Could you check a few things on this drawing? It's one solid part, dimensions in mm from its lowest x, y, z. A direction names the side the tool comes from. Coordinates: 2 decimals unless noted, no trailing zeros. Order: outer loops, then holes, each group sorted by start corner. A loop starts at its lowest first (then second) coordinate and runs counter-clockwise, first axis right, second up. Notation, with made-up numbers: (41.5, -31) - (63.5, -31) arc R19 ccw to (63.5, -13) - close; hole circle Ø10 at (62.5, -20). An arc over 180 degrees is marked (long way). Answer in a Markdown table with one row per item. Add a question column.
Item 1: I want a section at D-D (x = 37.5). Please give me the cut outline in (y, z).
Item 2: Will these pins go through, and if not, where does the flat tip stop? pin 1 Ø5 at (y, z) = (94.5, 3) entering from +X; pin 2 Ø5 at (x, z) = (37.5, 6) entering from -Y; pin 3 Ø2.5 at (x, y) = (125.38, 45.19) entering from -Z; pin 4 Ø8 at (x, y) = (75.5, 97.5) entering from -Z.
Item 3: I want a section at A-A (x = 85.19). Please give me the cut outline in (y, z).
Item 4: If I drill on line 1 along Y through (x, z) = (125.38, 3); line 2 along Y through (x, z) = (45.19, 3); line 3 along X through (y, z) = (122.5, 8), over which ranges is the centre line in solid material (lowest first)? Write a range as from..to.
Item 5: On a 3-axis mill with a long thin cutter (end or side, diameter ignored), from which of +Z, -Z, +X, -X, +Y, -Y can I reach the whole of each face in a straight line? I mean the marked faces 1, 2 and 3. Say none if no direction works.
Item 6: I want a section at C-C (z = 3.25). Count the separate pieces of the cut face and the enclosed holes in it, plus the area to 3 significant figures.
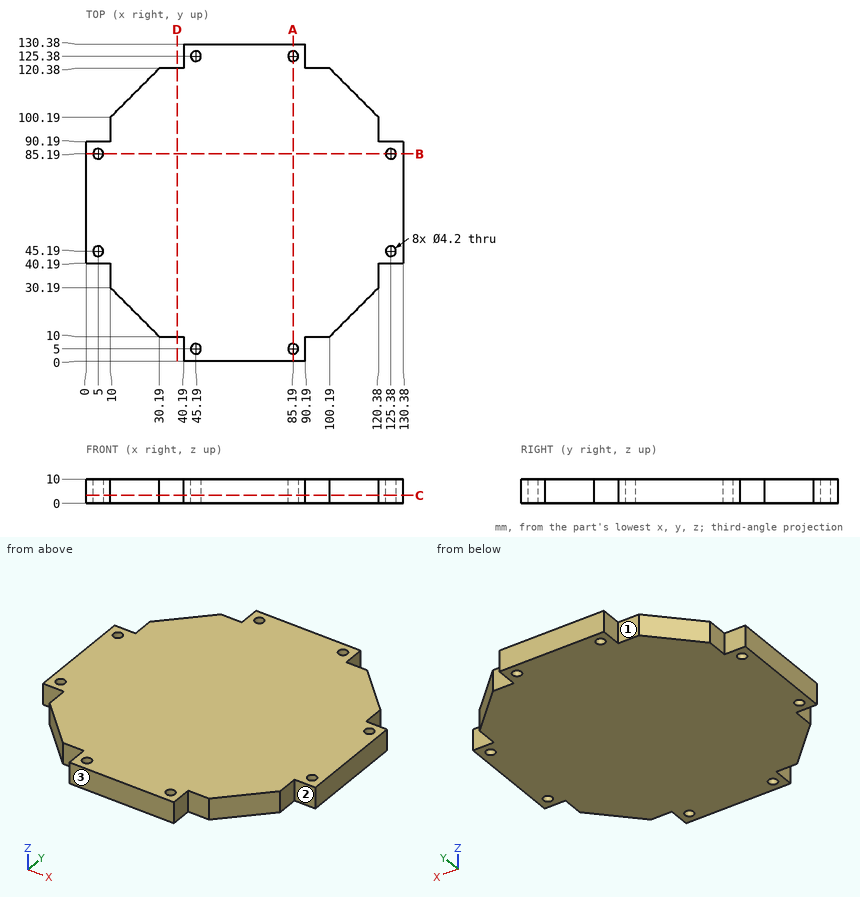
Values follow:
| question | item | result |
|---|---|---|
| 1 | outline | (10, 0) - (120.38, 0) - (120.38, 10) - (10, 10) - close |
| 2 | pin 1 | stops at x = 120.38 |
| 2 | pin 2 | stops at y = 10 |
| 2 | pin 3 | passes through |
| 2 | pin 4 | stops at z = 0 |
| 3 | outline | (0, 0) - (2.9, 0) - (2.9, 10) - (0, 10) - close; (7.1, 0) - (123.28, 0) - (123.28, 10) - (7.1, 10) - close; (127.48, 0) - (130.38, 0) - (130.38, 10) - (127.48, 10) - close |
| 4 | line 1 | y = 40.19..43.09, 47.29..83.09, 87.29..90.19 |
| 4 | line 2 | y = 0..2.9, 7.1..123.28, 127.48..130.38 |
| 4 | line 3 | x = 40.19..90.19 |
| 5 | face 1 | +Z, -Z, -X, +Y |
| 5 | face 2 | +Z, -Z, +X, -Y |
| 5 | face 3 | +Z, -Z, +X, -X, -Y |
| 6 | separate pieces | 1 |
| 6 | enclosed holes | 8 |
| 6 | area | 13,300 mm^2 |
